Input: part model. Units: mm. Frame: model coordinates. A direction names the side the tool comes from. Give positions to 0.01 mm unless a question says otherwise; leave off trailing zeros. Loops run counter-clockwise (first coordinate to the right, second up) from the corner with the lowest first, then second, coordinate; pieces in that order, holes last. Notation, with made-up numbers: (64.5, -19.5) - (110.5, -19.5) arc R14 ccw to (110.5, -5.5) - close; hole circle Ø10 at (80, 47). An arc over 180 degrees is marked (long way). Answer as a JSON object with one key per item and string values. Group by question number.
(1) Mould query, pull axis Y, two halves, no side actions, for faces 4 (the flat face through (-69, -11, 8)), 5 (the flat face through (4.3, 10.7, 28)), 6 (the flat face through (3.861, 10, 15)), 7 (the flat face through (-33, 46.556, 14)). Classes: +Y half, -Y half, draft (parallel to the pull), parting line (faces both ways), or undercut.
(2) Pin query (flat end, axial travel): P1, Ø0.6, axis at x = -69, y = 10.5, coming from the +Z side; P2, Ø10, axis at x = -26, y = 33, coming from the +Z side. Return the tip coordinate at first contact, or that it passes through.
(3) Section query B-B (x = -63). Return loops of the section in (y, z), plus the area to 3 significant figures.
(4) Access query for faces 1 (the flat face through (-69, 36.556, 18)), 2 (the flat face through (-70.139, 10.1, 7.6)), 3 (the flat face through (-60.139, -20, 4)). Directions: +Z, -Z, +X, -X, +Y, -Y. A direction counts if a zero-diameter tool reaches every point of the face in a straight line with its end or side. Return the directions, or none.
(5) Section query C-C (z = 20.75). Return loops of the section in (x, y).
(6) Material intervals for L1, parallel to X at y = 43.5, z = 26; L2, parallel to Y at x = -61, z = 13.5; L3, parallel to X at y = 7, z = 24.5, sorted ascending.
(7) Section query D-D (y = 20). Return loops of the section in (x, z).
(8) Section query A-A (z = 3.75). Return loops of the section in (x, y).
```python
from build123d import *

# Parameters (mm, degrees)
ESQUISSE1_W             = 76
ESQUISSE1_H             = 72
BOSS_EXTRU_1_DEPTH      = 2
ESQUISSE2_W             = 76
ESQUISSE2_H             = 72
ESQUISSE2_W_2           = 72
ESQUISSE2_H_2           = 68
BOSS_EXTRU_2_DEPTH      = 26
ESQUISSE3_W             = 8
ESQUISSE3_H             = 8
BOSS_EXTRU_3_DEPTH      = 4
ESQUISSE4_W             = 12.488308145
ESQUISSE4_H             = 8
ESQUISSE4_W_2           = 11.866165586
ESQUISSE4_H_2           = 11
ESQUISSE4_W_3           = 11.945061533
ESQUISSE4_H_3           = 14
ENL_V_MAT_EXTRU_1_DEPTH = 87.526649953


with BuildPart() as part:
    # Esquisse1 → Boss.-Extru.1 (new body)
    with BuildSketch(Plane.XY):
        with Locations((-32.138593491, 10.555760709)):
            Rectangle(ESQUISSE1_W, ESQUISSE1_H)
    extrude(amount=BOSS_EXTRU_1_DEPTH)

    # Esquisse2 → Boss.-Extru.2 (add)
    with BuildSketch(Plane.XY.offset(2)):
        with Locations((-32.138593491, 10.555760709)):
            Rectangle(ESQUISSE2_W, ESQUISSE2_H)
        with Locations((-32.138593491, 10.555760709)):
            Rectangle(ESQUISSE2_W_2, ESQUISSE2_H_2, mode=Mode.SUBTRACT)
    extrude(amount=BOSS_EXTRU_2_DEPTH)

    # Esquisse3 → Boss.-Extru.3 (add)
    with BuildSketch(Plane.XY.offset(2)):
        with Locations((-64.138593491, 40.555760709)):
            Rectangle(ESQUISSE3_W, ESQUISSE3_H)
        with Locations((-0.138593491, -19.444239291)):
            Rectangle(ESQUISSE3_W, ESQUISSE3_H)
        with Locations((-0.138593491, 40.555760709)):
            Rectangle(ESQUISSE3_W, ESQUISSE3_H)
        with Locations((-64.138593491, -19.444239291)):
            Rectangle(ESQUISSE3_W, ESQUISSE3_H)
    extrude(amount=BOSS_EXTRU_3_DEPTH)

    # Esquisse4 → Enlèv. mat.-Extru.1 (cut, through all)
    with BuildSketch(Plane.XY.offset(8)):
        with Locations((-68.655939158, -11.444239291)):
            Rectangle(ESQUISSE4_W, ESQUISSE4_H)
        with Locations((-68.344867878, 11.055760709)):
            Rectangle(ESQUISSE4_W_2, ESQUISSE4_H_2)
        with Locations((-70.945478816, 29.555760709)):
            Rectangle(ESQUISSE4_W_3, ESQUISSE4_H_3)
    extrude(amount=ENL_V_MAT_EXTRU_1_DEPTH, mode=Mode.SUBTRACT)


solid = part.part
```
Recorded:
{
 "1": {"face 4": "undercut", "face 5": "draft", "face 6": "undercut", "face 7": "+Y half"},
 "2": {"P1": "stops at z = 8", "P2": "stops at z = 2"},
 "3": {"outline": "(-25.44, 0) - (46.56, 0) - (46.56, 28) - (44.56, 28) - (44.56, 6) - (36.56, 6) - (36.56, 2) - (-15.44, 2) - (-15.44, 6) - (-23.44, 6) - (-23.44, 28) - (-25.44, 28) - close", "area": "312 mm^2"},
 "4": {"face 1": "+Z, -X", "face 2": "+Z, -Z, -X, +Y, -Y", "face 3": "+Z"},
 "5": {"outline": "(-70.14, -25.44) - (5.86, -25.44) - (5.86, 46.56) - (-70.14, 46.56) - (-70.14, 36.56) - (-68.14, 36.56) - (-68.14, 44.56) - (3.86, 44.56) - (3.86, -23.44) - (-68.14, -23.44) - (-68.14, -15.44) - (-70.14, -15.44) - close; (-70.14, -7.44) - (-68.14, -7.44) - (-68.14, 5.56) - (-70.14, 5.56) - close; (-70.14, 16.56) - (-68.14, 16.56) - (-68.14, 22.56) - (-70.14, 22.56) - close"},
 "6": {"L1": "x = -70.14 to -68.14, 3.86 to 5.86", "L2": "y = -25.44 to -23.44, 44.56 to 46.56", "L3": "x = 3.86 to 5.86"},
 "7": {"outline": "(-70.14, 0) - (5.86, 0) - (5.86, 28) - (3.86, 28) - (3.86, 2) - (-68.14, 2) - (-68.14, 28) - (-70.14, 28) - close"},
 "8": {"outline": "(-70.14, -25.44) - (5.86, -25.44) - (5.86, 46.56) - (-70.14, 46.56) - close; hole (-68.14, -15.44) - (-60.14, -15.44) - (-60.14, -23.44) - (-4.14, -23.44) - (-4.14, -15.44) - (3.86, -15.44) - (3.86, 36.56) - (-4.14, 36.56) - (-4.14, 44.56) - (-60.14, 44.56) - (-60.14, 36.56) - (-68.14, 36.56) - close"}
}
